Part print with two shaded views. Sizes in mm from the minimum x, y, z corner. A direction names the side the tool comes from. Give positions to 0.01 mm unless a question says otherwise; leave off trailing zeros. Loops run counter-clockwise (first coordinate to the right, second up) from the corner with the lowest first, then second, coordinate; pieces in that order, holes last. Notation, with made-up numbers: M 84.25,84 L 143.25,84 A6 cw 143.25,91 Z; hole C 49.5,19.25 d11. An arc over 180 degrees is marked long. Answer in a Markdown table with one row per item.
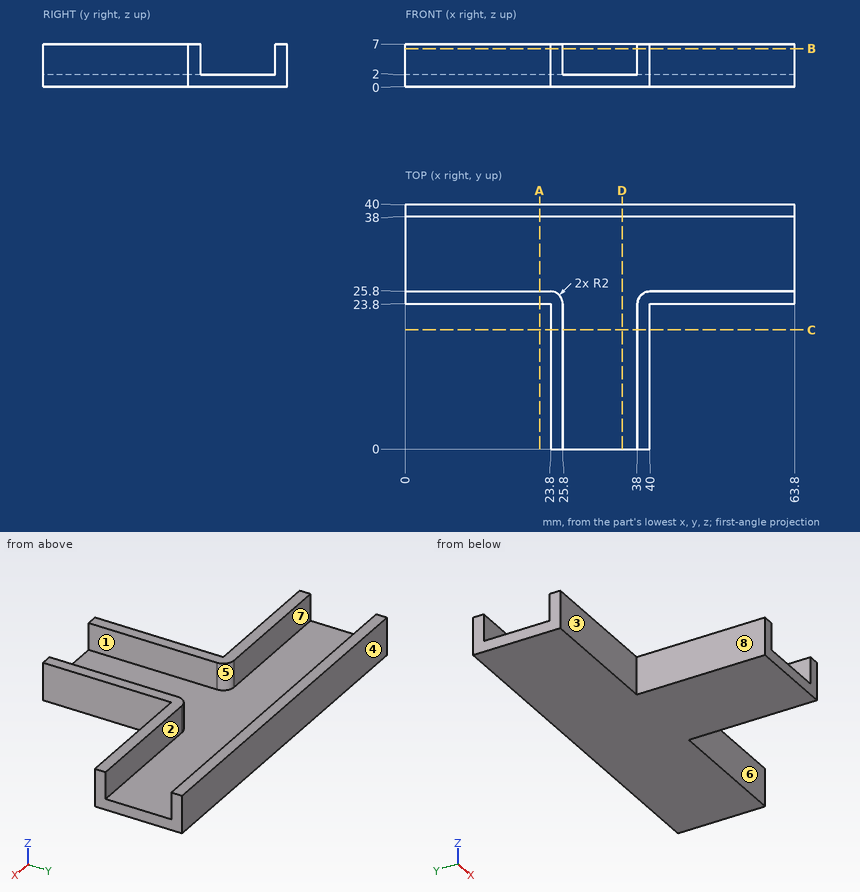
Q1. Drop flat-ended pins along their axis: pin 1 (4 mm diameter, centred on x = 43.5, y = 21, fed in from +Z); pin 2 (2 mm diameter, centred on x = 7.5, z = 3.5, fed in from -Y); pin 3 (2 mm diameter, centred on y = 16.5, z = 4, fed in from +X). Give the stop position or say it passes through.
Reported:
| item | result |
|---|---|
| pin 1 | through |
| pin 2 | y = 23.8 |
| pin 3 | x = 40 |
Q2. Mould opens along Y. For the marked faces 1, 2 and 3 say: released by +Y, released by -Y, zero draft, split by the parting line, or undercut.
Reported:
| item | result |
|---|---|
| face 1 | zero draft |
| face 2 | undercut |
| face 3 | released by -Y |
Q3. Saw through at A-A (x = 22). Give the cut face in (y, z), and give its area (3 significant figures).
Reported:
| item | result |
|---|---|
| outline | M 23.8,0 L 40,0 L 40,7 L 38,7 L 38,2 L 25.8,2 L 25.8,7 L 23.8,7 Z |
| area | 52.4 mm² |
Q4. Saw through at D-D (x = 35.5). Give the cut face in (y, z), and give its area (3 significant figures).
Reported:
| item | result |
|---|---|
| outline | M 0,0 L 40,0 L 40,7 L 38,7 L 38,2 L 0,2 Z |
| area | 90.0 mm² |
Q5. Probe probe 1 along Y at (x, z) = (43, 3.75); probe 2 along Y at (x, z) = (31.5, 5). List the from-to ranges inside material, lowest first.
Reported:
| item | result |
|---|---|
| probe 1 | 23.8 to 25.8, 38 to 40 |
| probe 2 | 38 to 40 |
Q6. 3-axis set-ups, long thin cutter, end or side, ignore diameter. For the marked faces 4, 5, 6, 7 and 8: which of +Z, -Z, +X, -X, +Y, -Y reach the whole face in a straight line?
Reported:
| item | result |
|---|---|
| face 4 | +Z, -Z, +X, -X, +Y |
| face 5 | +Z |
| face 6 | +Z, -Z, +X, -Y |
| face 7 | +Z, +X, -X |
| face 8 | +Z, -Z, -X, -Y |
Q7. Saw through at B-B (z = 6.25). Give the cut face in (x, y).
Reported:
| item | result |
|---|---|
| outline | M 0,23.8 L 23.8,23.8 L 23.8,0 L 25.8,0 L 25.8,23.8 A2 ccw 23.8,25.8 L 0,25.8 Z; M 0,38 L 63.8,38 L 63.8,40 L 0,40 Z; M 38,0 L 40,0 L 40,23.8 L 63.8,23.8 L 63.8,25.8 L 40,25.8 A2 ccw 38,23.8 Z |
